from build123d import *

# Parameters (mm, degrees)
CONVERTED1_START         = 177.799999714
CONVERTED1_DEPTH         = 177.799999714
CONVERTED1_2_OUTLINE_W   = 67.310094833
CONVERTED1_2_OUTLINE_H   = 144.784152508
CONVERTED1_2_OUTLINE_H_2 = 55.875837803
CONVERTED1_2_OUTLINE_W_2 = 67.310005426
CONVERTED1_2_DEPTH       = 177.799999714
CONVERTED1_START_2       = 125.335559249
CONVERTED1_3_OUTLINE_W   = 67.310094833
CONVERTED1_3_OUTLINE_H   = 78.740000725
CONVERTED1_3_OUTLINE_W_2 = 67.310005426
CONVERTED1_3_DEPTH       = 52.464440465
CONVERTED1_START_3       = -1
CONVERTED1_4_DEPTH       = 1292
SKETCH1_W                = 67.310005426
SKETCH1_H                = 144.784152508
SKETCH1_H_2              = 55.875837803
SKETCH1_W_2              = 67.310094833
BOSS_EXTRUDE1_DEPTH      = 100


with BuildPart() as part:
    # Converted1: read off the stored shape, not the designer's step
    # Converted1 outline → Converted1 (new body)
    with BuildSketch(Plane(origin=(0, 0, 0), x_dir=(1, 0, 0), z_dir=(0, 1, 0)).offset(CONVERTED1_START)):
        Polygon((1223.009943962, -165.100008249), (1223.009943962, 0), (791.113138199, 0), (791.113138199, -101.599998772), (486.313134432, -101.599998772), (486.313134432, 0), (67.310005426, 0), (67.310005426, -165.100008249), (0, -165.100008249), (0, -444.499999285), (67.310005426, -444.499999285), (67.310005426, -520.699977875), (486.313134432, -520.699977875), (486.313134432, -457.199990749), (791.113138199, -457.199990749), (791.113138199, -520.699977875), (1223.009943962, -520.699977875), (1223.009943962, -444.499999285), (1290.320038795, -444.499999285), (1290.320038795, -165.100008249), align=None)
        Polygon((515.501916409, -226.575806737), (518.159985542, -260.349988937), (515.501916409, -294.124186039), (507.593095303, -327.066779137), (494.628280401, -358.366549015), (476.926743984, -387.25283742), (454.924374819, -413.014382124), (429.162800312, -435.016751289), (400.27654171, -452.718287706), (368.976742029, -465.683102608), (336.034178734, -473.591923714), (302.259981632, -476.249992847), (268.485784531, -473.591923714), (235.543236136, -465.683102608), (204.243451357, -452.718287706), (175.357162952, -435.016751289), (149.59564805, -413.014382124), (127.593204379, -387.25283742), (109.891682863, -358.366549015), (96.926905215, -327.066779137), (89.018076658, -294.124186039), (86.360000074, -260.349988937), (89.018076658, -226.575806737), (96.926905215, -193.633243442), (109.891682863, -162.333458662), (127.593204379, -133.447170258), (149.59564805, -107.685647905), (175.357162952, -85.683234036), (204.243451357, -67.98170507), (235.543236136, -55.016901344), (268.485784531, -47.108106315), (302.259981632, -44.449992478), (336.034178734, -47.108106315), (368.976742029, -55.016901344), (400.27654171, -67.98170507), (429.162800312, -85.683234036), (454.924374819, -107.685647905), (476.926743984, -133.447170258), (494.628280401, -162.333458662), (507.593095303, -193.633243442), align=None, mode=Mode.SUBTRACT)
        Polygon((1054.776668549, -55.016901344), (1086.076498032, -67.98170507), (1114.962816238, -85.683234036), (1140.724420547, -107.685647905), (1162.726759911, -133.447170258), (1180.428385735, -162.333458662), (1193.39299202, -193.633243442), (1201.301813126, -226.575806737), (1203.959941864, -260.349988937), (1201.301813126, -294.124186039), (1193.39299202, -327.066779137), (1180.428385735, -358.366549015), (1162.726759911, -387.25283742), (1140.724420547, -413.014382124), (1114.962816238, -435.016751289), (1086.076498032, -452.718287706), (1054.776668549, -465.683102608), (1021.834254265, -473.591923714), (988.060057163, -476.249992847), (954.285860062, -473.591923714), (921.343266964, -465.683102608), (890.043437481, -452.718287706), (861.157119274, -435.016751289), (835.395634174, -413.014382124), (813.393175602, -387.25283742), (795.691668987, -358.366549015), (782.726883888, -327.066779137), (774.818062782, -294.124186039), (772.159993649, -260.349988937), (774.818062782, -226.575806737), (782.726883888, -193.633243442), (795.691668987, -162.333458662), (813.393175602, -133.447170258), (835.395634174, -107.685647905), (861.157119274, -85.683234036), (890.043437481, -67.98170507), (921.343266964, -55.016901344), (954.285860062, -47.108106315), (988.060057163, -44.449992478), (1021.834254265, -47.108106315), align=None, mode=Mode.SUBTRACT)
    extrude(amount=CONVERTED1_DEPTH)



with BuildPart() as body_2:
    # Converted1 2 outline → Converted1 2 (new body)
    with BuildSketch(Plane(origin=(0, 0, 0), x_dir=(1, 0, 0), z_dir=(0, 1, 0))):
        with Locations((1256.664991378, -237.492084503)):
            Rectangle(CONVERTED1_2_OUTLINE_W, CONVERTED1_2_OUTLINE_H)
        with Locations((1256.664991378, -416.562080384)):
            Rectangle(CONVERTED1_2_OUTLINE_W, CONVERTED1_2_OUTLINE_H_2)
        with Locations((33.655002713, -237.492084503)):
            Rectangle(CONVERTED1_2_OUTLINE_W_2, CONVERTED1_2_OUTLINE_H)
        with Locations((33.655002713, -416.562080384)):
            Rectangle(CONVERTED1_2_OUTLINE_W_2, CONVERTED1_2_OUTLINE_H_2)
    extrude(amount=CONVERTED1_2_DEPTH)


with BuildPart() as part_1:
    add(part.part)

    add(body_2.part)  # Converted1 3 merges body 2
    # Converted1 3 outline → Converted1 3 (add)
    with BuildSketch(Plane(origin=(0, 0, 0), x_dir=(1, 0, 0), z_dir=(0, 1, 0)).offset(CONVERTED1_START_2)):
        with Locations((1256.664991378, -349.25416112)):
            Rectangle(CONVERTED1_3_OUTLINE_W, CONVERTED1_3_OUTLINE_H)
        with Locations((33.655002713, -349.25416112)):
            Rectangle(CONVERTED1_3_OUTLINE_W_2, CONVERTED1_3_OUTLINE_H)
    extrude(amount=CONVERTED1_3_DEPTH)

    # Converted1 4 outline → Converted1 4 (cut)
    with BuildSketch(Plane.YZ.offset(CONVERTED1_START_3)):
        Polygon((125.335559249, 388.624161482), (125.335559249, 309.884160757), (172.469392419, 350.206673145), align=None)
    extrude(amount=CONVERTED1_4_DEPTH, mode=Mode.SUBTRACT)

    # Sketch1 → Boss-Extrude1 (add)
    with BuildSketch(Plane.XZ):
        with Locations((33.655002713, 237.492084503)):
            Rectangle(SKETCH1_W, SKETCH1_H)
        with Locations((33.655002713, 416.562080384)):
            Rectangle(SKETCH1_W, SKETCH1_H_2)
        with Locations((1256.664991378, 416.562080384)):
            Rectangle(SKETCH1_W_2, SKETCH1_H_2)
        with Locations((1256.664991378, 237.492084503)):
            Rectangle(SKETCH1_W_2, SKETCH1_H)
    extrude(amount=BOSS_EXTRUDE1_DEPTH)


solid = part_1.part
The model under review builds one solid part; all positions refer to its coordinate system, in mm. A direction names the side the tool comes from. Round coordinates to 2 decimals unless told otherwise and drop trailing zeros. Loops run counter-clockwise (first coordinate to the right, second up) from the corner with the lowest first, then second, coordinate; pieces in that order, holes last. Notation, with made-up numbers: (55.25, 50.25) -> (114.25, 50.25) arc R12 ccw to (114.25, 55.25) -> close; hole circle Ø10 at (-11, -21). An arc over 180 degrees is marked (long way). One line per question, with ' | ' between items. Start each with the question number.
Item 1: Add section A-A, the plane y = -28.5. Write out the cut boundary in (x, z).
Item 2: Add section D-D, the plane y = 144.5. Write out the cut boundary in (x, z), then the cut area to 3 significant figures.
Item 3: Draft analysis for pull direction Z (two halves, no side actions). For faces 1 (the face through (1005.2, 265.5, 474.9)), 2 (the face through (280, 265, 0)), 3 (the face through (274, 265, 520.7)), 4 (the face through (103.32, 265.46, 178.2)), state which applies: +Z half, -Z half, draft (parallel to the pull), parting line (faces both ways), or undercut.
Item 4: Wall thickness on line 1 along X through (y, z) = (269, 89); line 2 along X through (y, z) = (99, 304); line 3 along X through (y, z) = (308, 324): over which ranges is each line inside the solid? List them lowest first. Write a range as [from, to].
Item 5: Add section C-C, the plane y = 253. Count the separate pieces of the cut face and the enclosed holes in it, then the cut area to 3 significant figures.
Item 6: Machinability: for faces 5 (the face through (285.1, 265.5, 45.8)), 6 (the face through (791.113, 265, 50)), 7 (the face through (791.113, 265, 489)), which of the approach directions +Z, -Z, +X, -X, +Y, -Y give a long, thin tool a straight path to every point of the face, cutting with its end or side? Answer none if there is none.
Item 7: Add section B-B, the plane x = 216. Write out the cut boundary in (y, z).
Return value:
1) outline: (0, 165.1) -> (67.31, 165.1) -> (67.31, 309.88) -> (0, 309.88) -> close; (0, 388.62) -> (67.31, 388.62) -> (67.31, 444.5) -> (0, 444.5) -> close; (1223.01, 165.1) -> (1290.32, 165.1) -> (1290.32, 309.88) -> (1223.01, 309.88) -> close; (1223.01, 388.62) -> (1290.32, 388.62) -> (1290.32, 444.5) -> (1223.01, 444.5) -> close
2) outline: (0, 165.1) -> (67.31, 165.1) -> (67.31, 326.28) -> (0, 326.28) -> close; (0, 373) -> (67.31, 373) -> (67.31, 444.5) -> (0, 444.5) -> close; (1223.01, 165.1) -> (1290.32, 165.1) -> (1290.32, 326.28) -> (1223.01, 326.28) -> close; (1223.01, 373) -> (1290.32, 373) -> (1290.32, 444.5) -> (1223.01, 444.5) -> close | area: 31,300 mm2
3) face 1: undercut | face 2: -Z half | face 3: +Z half | face 4: undercut
4) line 1: x = [67.31, 171.47], [433.05, 486.31], [791.11, 857.27], [1118.85, 1223.01] | line 2: x = [0, 67.31], [1223.01, 1290.32] | line 3: x = [0, 96.19], [508.33, 781.99], [1194.13, 1290.32]
5) separate pieces: 1 | enclosed holes: 2 | area: 297,000 mm2
6) face 5: +Y, -Y | face 6: -Z, +Y, -Y | face 7: +Z, +Y, -Y
7) outline: (177.8, 0) -> (355.6, 0) -> (355.6, 63.11) -> (177.8, 63.11) -> close; (177.8, 457.59) -> (355.6, 457.59) -> (355.6, 520.7) -> (177.8, 520.7) -> close
